Part print with two shaded views. Sizes in mm from the minimum x, y, z corner. A direction names the side the tool comes from. Round coordinates to 2 decimals unless told otherwise and drop trailing zeros. Loops run counter-clockwise (first coordinate to the right, second up) from the corner with the lowest first, then second, coordinate; pieces in that order, holes last. Notation, with made-up numbers: (59, -6) -> (76, -6) arc R29 ccw to (76, 26) -> close; hole circle Ø8 at (59.5, 35). An arc over 180 degrees is marked (long way). Put each result on its own line as item: value. Start each with the question number.
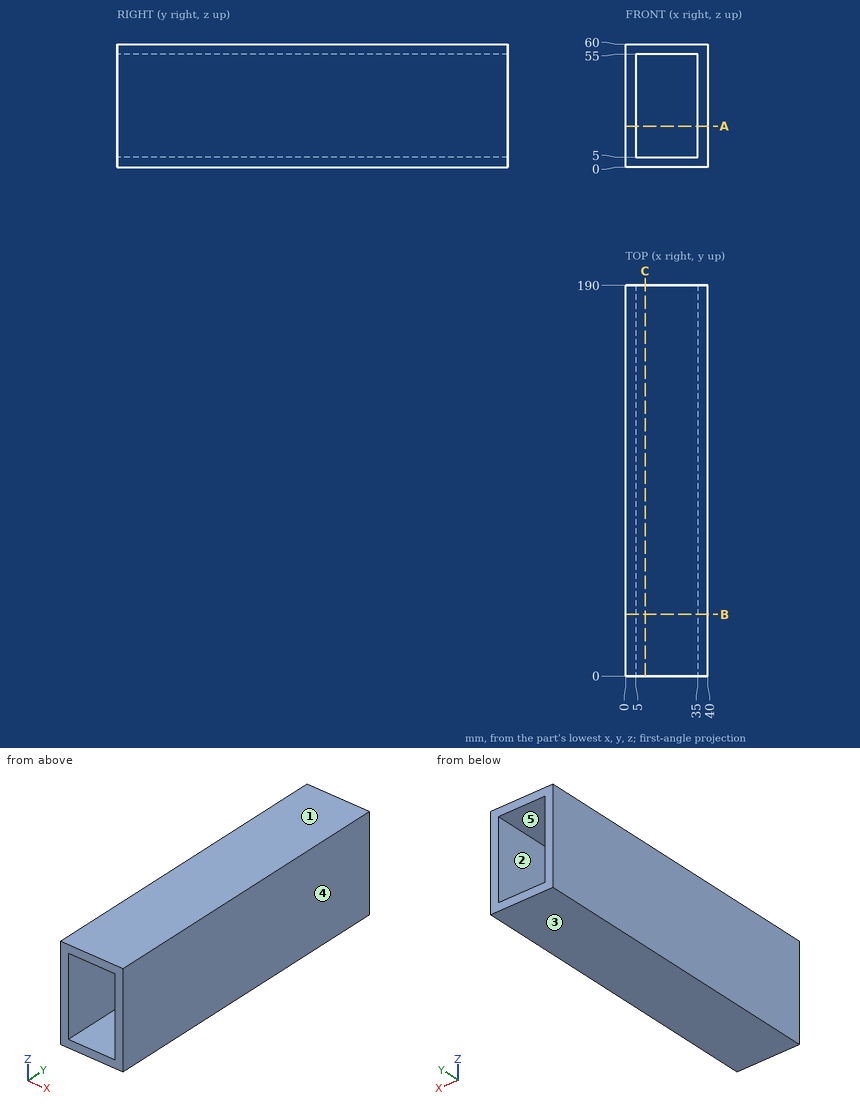
Item 1: 3-axis set-ups, long thin cutter, end or side, ignore diameter. For the marked faces 1 and 2: which of +Z, -Z, +X, -X, +Y, -Y reach the whole face in a straight line?
Item 2: Pull direction X, two halves, no side cores. Call the marked faces 3, 4 and 5: +X half, -X half, draft (parallel to the pull), parting line (faces both ways), or undercut.
Item 3: Cut at A-A on z = 20. Write the cut outline in (x, y).
Item 4: Cut at B-B on y = 30. Write the cut outline in (x, z).
Item 5: Cut at C-C on x = 9.5. Write the cut outline in (y, z).
Item 6: Drop a flat-ended pin along its axis: pin 1 (8 mm diameter, centred on x = 10.5, z = 48, fed in from +Y). Give the stop position or say it passes through.
Item 7: Wall check: line 1 (X direction, y = 92, z = 42); line 2 (Z direction, x = 33.5, y = 166). Give the ranges that are in metal, low to high. Write a range as from..to.
Ans:
1. face 1: +Z, +X, -X, +Y, -Y
1. face 2: +Y, -Y
2. face 3: draft
2. face 4: +X half
2. face 5: undercut
3. outline: (0, 0) -> (5, 0) -> (5, 190) -> (0, 190) -> close; (35, 0) -> (40, 0) -> (40, 190) -> (35, 190) -> close
4. outline: (0, 0) -> (40, 0) -> (40, 60) -> (0, 60) -> close; hole (5, 5) -> (35, 5) -> (35, 55) -> (5, 55) -> close
5. outline: (0, 0) -> (190, 0) -> (190, 5) -> (0, 5) -> close; (0, 55) -> (190, 55) -> (190, 60) -> (0, 60) -> close
6. pin 1: passes through
7. line 1: x = 0..5, 35..40
7. line 2: z = 0..5, 55..60
